```python
from build123d import *

# Parameters (mm, degrees)
SKETCH1_W                                       = 45
SKETCH1_H                                       = 25
BOSS_EXTRUDE1_DEPTH                             = 3
CSK_FOR_M2_FLAT_HEAD_MACHINE_SCREW1_D           = 2.4
CSK_FOR_M2_FLAT_HEAD_MACHINE_SCREW1_CSINK_D     = 4.4
CSK_FOR_M2_FLAT_HEAD_MACHINE_SCREW1_CSINK_ANGLE = 90
CSK_FOR_M2_FLAT_HEAD_MACHINE_SCREW2_D           = 2.4
CSK_FOR_M2_FLAT_HEAD_MACHINE_SCREW2_CSINK_D     = 4.4
CSK_FOR_M2_FLAT_HEAD_MACHINE_SCREW2_CSINK_ANGLE = 90


with BuildPart() as part:
    # Sketch1 → Boss-Extrude1 (new body)
    with BuildSketch(Plane.XY):
        Rectangle(SKETCH1_W, SKETCH1_H)
    extrude(amount=BOSS_EXTRUDE1_DEPTH)

    # CSK for M2 Flat Head Machine Screw1 (through all)
    with Locations(Plane.XY.offset(3)):
        with Locations((-19.5, 9), (19.5, 9), (19.5, -9), (-19.5, -9)):
            CounterSinkHole(CSK_FOR_M2_FLAT_HEAD_MACHINE_SCREW1_D / 2, CSK_FOR_M2_FLAT_HEAD_MACHINE_SCREW1_CSINK_D / 2, counter_sink_angle=CSK_FOR_M2_FLAT_HEAD_MACHINE_SCREW1_CSINK_ANGLE)

    # CSK for M2 Flat Head Machine Screw2 (through all)
    with Locations(Plane(origin=(0, 0, 0), x_dir=(-1, 0, 0), z_dir=(0, 0, -1))):
        with Locations((12.8, 0)):
            CounterSinkHole(CSK_FOR_M2_FLAT_HEAD_MACHINE_SCREW2_D / 2, CSK_FOR_M2_FLAT_HEAD_MACHINE_SCREW2_CSINK_D / 2, counter_sink_angle=CSK_FOR_M2_FLAT_HEAD_MACHINE_SCREW2_CSINK_ANGLE)


solid = part.part
```
The listing builds one solid part. Answer for the finished solid, in the listing's coordinates (mm). Give positions to 0.01 mm unless a question says otherwise; leave off trailing zeros. Order: outer loops, then holes, each group sorted by start corner. A loop starts at its lowest first (then second) coordinate and runs counter-clockwise, first axis right, second up. Notation, with made-up numbers: (13, 89.25) -> (49, 89.25) arc R30 ccw to (49, 128.25) -> close; hole circle Ø7 at (60, -25). An arc over 180 degrees is marked (long way). One line per item, written item: value.
1) Find section B-B, the plane y = -9. Determine the outline of the cut face in (x, z), plus the area to 3 significant figures.
Reported:
outline: (-22.5, 0) -> (-20.7, 0) -> (-20.7, 2) -> (-21.7, 3) -> (-22.5, 3) -> close; (-18.3, 0) -> (18.3, 0) -> (18.3, 2) -> (17.3, 3) -> (-17.3, 3) -> (-18.3, 2) -> close; (20.7, 0) -> (22.5, 0) -> (22.5, 3) -> (21.7, 3) -> (20.7, 2) -> close
area: 119 mm^2
2) Find section D-D, the plane x = -12.8. Determine the outline of the cut face in (y, z), plus the area to 3 significant figures.
Reported:
outline: (-12.5, 0) -> (-2.2, 0) -> (-1.2, 1) -> (-1.2, 3) -> (-12.5, 3) -> close; (1.2, 1) -> (2.2, 0) -> (12.5, 0) -> (12.5, 3) -> (1.2, 3) -> close
area: 66.8 mm^2
3) A flat-ended cylindrical pin translates along its axis: P1, Ø4, axis at x = -12.8, y = 0, coming from the -Z side. Find the tip coordinate at first contact, or state that the pin passes through.
Reported:
P1: stops at z = 0.2
4) Find section A-A, the plane y = 0. Determine the outline of the cut face in (x, z).
Reported:
outline: (-22.5, 0) -> (-15, 0) -> (-14, 1) -> (-14, 3) -> (-22.5, 3) -> close; (-11.6, 1) -> (-10.6, 0) -> (22.5, 0) -> (22.5, 3) -> (-11.6, 3) -> close
5) Determine the mould class of faces 1 (the flat face through (0, -12.5, 1)), 2 (the cylindrical face through (-14, 0, 2)), 3 (the flat face through (22.5, 0, 1)) for opening direction X: pulls with the +X half, pulls with the -X half, needs draft (parallel to the pull), parting line crosses it, or undercut.
Reported:
face 1: needs draft
face 2: undercut
face 3: pulls with the +X half
6) Find section C-C, the plane x = 19.5. Determine the outline of the cut face in (y, z), plus the area to 3 significant figures.
Reported:
outline: (-12.5, 0) -> (-10.2, 0) -> (-10.2, 2) -> (-11.2, 3) -> (-12.5, 3) -> close; (-7.8, 0) -> (7.8, 0) -> (7.8, 2) -> (6.8, 3) -> (-6.8, 3) -> (-7.8, 2) -> close; (10.2, 0) -> (12.5, 0) -> (12.5, 3) -> (11.2, 3) -> (10.2, 2) -> close
area: 58.6 mm^2
7) Find the intervals of material crossed by line 1 (X direction, y = -9, z = 0.45); line 2 (Y direction, x = -19.5, z = 0.7); line 3 (X direction, y = 0, z = 2.35), in increasing order.
Reported:
line 1: x = -22.5 to -20.7, -18.3 to 18.3, 20.7 to 22.5
line 2: y = -12.5 to -10.2, -7.8 to 7.8, 10.2 to 12.5
line 3: x = -22.5 to -14, -11.6 to 22.5
